The listing builds one solid part. Answer for the finished solid, in the listing's coordinates (mm). Face numbers are marked on the shaded views. A direction names the side the tool comes from. Coordinates: 2 decimals unless noted, no trailing zeros. Order: outer loops, then holes, each group sorted by start corner. A loop starts at its lowest first (then second) coordinate and runs counter-clockwise, first axis right, second up. Notation, with made-up numbers: (15.5, -34.5) - (69.5, -34.5) arc R14 cw to (69.5, -7.5) - close; hole circle Ø3 at (5.5, 34.5). An arc over 180 degrees is marked (long way). One line per item, written item: value. Start each with the question number.
Autodesk Inventor part; units mm, degrees
ref_plane "YZ Plane" through (0, 0, 0) normal (1, 0, 0) x (0, 1, 0)
ref_plane "XZ Plane" through (0, 0, 0) normal (0, 1, 0) x (-1, 0, 0)
ref_plane "XY Plane" through (0, 0, 0) normal (0, 0, 1) x (1, 0, 0)
sketch "Sketch1" plane through (0, 0, 0) normal (0, 0, 1) x (1, 0, 0)
  line L0 (0, 0) -> (175, 0)
  line L1 (175, 0) -> (175, 40)
  line L2 (175, 40) -> (0, 40)
  line L3 (0, 40) -> (0, 0)
  dimension "d0" = 175
  dimension "d1" = 40
extrude "Plate1" add sketch "Sketch1" along normal blind 3
sketch "Sketch2" plane through (0, 3, 3) normal (0, -1, 0) x (1, 0, 0)
  line L0 (175, 0) -> (0, 0)
  line L1 (0, 0) -> (0, -25)
  line L2 (0, -25) -> (175, -25)
  line L3 (175, -25) -> (175, 0)
edge flange "Flange1" height 25 angle 90 thickness 3 bend radius 0.5 thickness toward (0, -1, 0) relief tear relief width 3 relief depth 1.5 edges at (87.5, 0, 0) wall of the first edge with corners at (175, 3, 3) (0, 3, 3) (0, 3, -22) (175, 3, -22)
bend "Bend1"
corner "Corner1"
hole "Hole3" at (146, 25, 3) direction (0, 0, -1) diameter 5 end through all
hole "Hole4" at (86, 25, 3) direction (0, 0, -1) diameter 5 end through all
hole "Hole5" at (15, 3, -12) direction (0, -1, 0) diameter 5 end through all
equation "\"d38\" = Thickness"
equation "\"d47\" = Thickness"
equation "\"d56\" = Thickness"
equation "\"d3\" = BendReliefWidth"
equation "\"d4\" = BendReliefDepth"
equation "\"d5\" = MinimumRemnant"
equation "\"d6\" = BendRadius"
equation "\"d10\" = CornerReliefSize"
equation "\"d11\" = GapSize"
equation "\"d12\" = JacobiRadiusSize"
equation "\"BendRadius\" = Thickness"
equation "\"BendReliefWidth\" = Thickness"
equation "\"BendReliefDepth\" = 0.5 * Thickness"
equation "\"CornerReliefSize\" = 4 * Thickness"
equation "\"MinimumRemnant\" = 2 * Thickness"
equation "\"TransitionRadius\" = BendRadius"
equation "\"JacobiRadiusSize\" = BendRadius"
equation "\"GapSize\" = Thickness"
equation "\"d2\" = BendRadius"
properties part number "endcapOptionLeftAngle" material "Aluminum 6061"
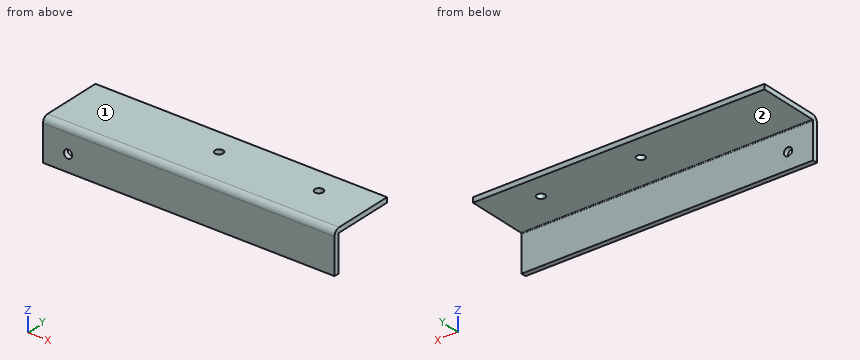
(1) Flat-ended cylindrical pins translate along their axes: pin 1 Ø10 at (x, y) = (72, 15.5) entering from -Z; pin 2 Ø4.5 at (x, y) = (146, 25) entering from +Z; pin 3 Ø12 at (x, z) = (150, -11) entering from +Y. Find the tip coordinate at first contact, or state that the pin passes through.
(2) The part is cut by section B-B on z = -12. Determine the outline of the cut face in (x, y).
(3) The part is cut by section A-A on y = 25. Determine the outline of the cut face in (x, z).
(4) For the marked faces 1 and 2, determine the directions among +Z, -Z, +X, -X, +Y, -Y from which every point of the face is accessible in a straight line to the end or side of a thin tool.
(5) Consider probe 1 along X at (y, z) = (25, 1.6); probe 2 along X at (y, z) = (1, -12); probe 3 along Z at (x, y) = (11, 34). Determine where each line is inside the solid, lowest interval first.
(6) The part is cut by section D-D on x = 95. Determine the outline of the cut face in (y, z).
(7) The part is cut by section C-C on x = 146. Determine the outline of the cut face in (y, z).
Completed:
1. pin 1: stops at z = 0
1. pin 2: passes through
1. pin 3: stops at y = 3
2. outline: (0, 0) - (12.5, 0) - (12.5, 3) - (0, 3) - close; (17.5, 0) - (175, 0) - (175, 3) - (17.5, 3) - close
3. outline: (0, 0) - (83.5, 0) - (83.5, 3) - (0, 3) - close; (88.5, 0) - (143.5, 0) - (143.5, 3) - (88.5, 3) - close; (148.5, 0) - (175, 0) - (175, 3) - (148.5, 3) - close
4. face 1: +Z, +X, -X, +Y, -Y
4. face 2: -Z, +X, -X, +Y
5. probe 1: x = 0 to 83.5, 88.5 to 143.5, 148.5 to 175
5. probe 2: x = 0 to 12.5, 17.5 to 175
5. probe 3: z = 0 to 3
6. outline: (0, -22) - (3, -22) - (3, -0.5) arc R0.5 cw to (3.5, 0) - (40, 0) - (40, 3) - (3.5, 3) arc R3.5 ccw to (0, -0.5) - close
7. outline: (0, -22) - (3, -22) - (3, -0.5) arc R0.5 cw to (3.5, 0) - (22.5, 0) - (22.5, 3) - (3.5, 3) arc R3.5 ccw to (0, -0.5) - close; (27.5, 0) - (40, 0) - (40, 3) - (27.5, 3) - close
